```python
from build123d import *

# Parameters (mm, degrees)
ESQUISSE2_W                     = 381
ESQUISSE2_H                     = 95.25
BOSS_EXTRU_1_DEPTH              = 6.35
ESQUISSE3_W                     = 38.1
ESQUISSE3_H                     = 6.35
BOSS_EXTRU_2_DEPTH              = 6.35
ESQUISSE4_W                     = 38.1
ESQUISSE4_H                     = 6.35
ENL_V_MAT_EXTRU_1_DEPTH         = 6.35
R_P_TITION_LIN_AIRE1_COUNT      = 4
R_P_TITION_LIN_AIRE1_PITCH      = 76.2
R_P_TITION_LIN_AIRE1_COUNT_DIR2 = 2
R_P_TITION_LIN_AIRE1_PITCH_DIR2 = 88.9


with BuildPart() as part:
    # Esquisse2 → Boss.-Extru.1 (new body)
    with BuildSketch(Plane(origin=(0, 0, 0), x_dir=(1, 0, 0), z_dir=(0, 1, 0))):
        Rectangle(ESQUISSE2_W, ESQUISSE2_H)
    extrude(amount=BOSS_EXTRU_1_DEPTH)

    # Esquisse3 → Boss.-Extru.2 (add)
    with BuildSketch(Plane(origin=(190.5, 0, 0), x_dir=(0, 0, -1), z_dir=(1, 0, 0))):
        with Locations((0, 3.175)):
            Rectangle(ESQUISSE3_W, ESQUISSE3_H)
    boss_extru_2 = extrude(amount=BOSS_EXTRU_2_DEPTH)

    # Esquisse4 → Enlèv. mat.-Extru.1 (cut)
    with BuildSketch(Plane(origin=(0, 0, -47.625), x_dir=(-1, 0, 0), z_dir=(0, 0, -1))):
        with Locations((-114.3, 3.175)):
            Rectangle(ESQUISSE4_W, ESQUISSE4_H)
    enl_v_mat_extru_1 = extrude(amount=-ENL_V_MAT_EXTRU_1_DEPTH, mode=Mode.SUBTRACT)

    # Répétition linéaire1: Enl_v. mat.-Extru.1 4 × 2
    with Locations(*[(-i * R_P_TITION_LIN_AIRE1_PITCH, 0, j * R_P_TITION_LIN_AIRE1_PITCH_DIR2) for i in range(R_P_TITION_LIN_AIRE1_COUNT) for j in range(R_P_TITION_LIN_AIRE1_COUNT_DIR2) if (i, j) != (0, 0)]):
        add(enl_v_mat_extru_1, mode=Mode.SUBTRACT)

    # Symétrie1: Boss.-Extru.2 across plane
    add(boss_extru_2.mirror(Plane(origin=(0, 0, 0), x_dir=(0, 0, 1), z_dir=(1, 0, 0))))


solid = part.part
```
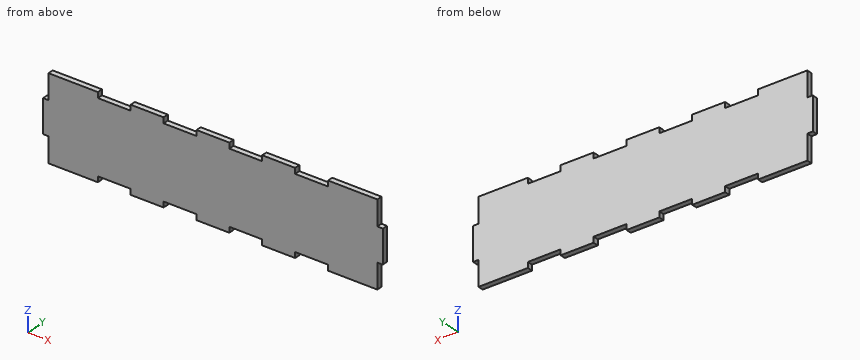
Input: part model. Units: mm. Frame: model coordinates. Give positions to 0.01 mm unless a question says otherwise; leave off trailing zeros. Order: outer loops, then holes, each group sorted by start corner. A loop starts at its lowest first (then second) coordinate and runs counter-clockwise, first axis right, second up. Notation, with made-up numbers: (11, -14.75) - (69, -14.75) arc R9 cw to (69, -0.75) - close; hole circle Ø11 at (-23, 37.25). An arc over 180 degrees is marked (long way). Use a Markdown table: item, result.
(1) Line query: line 1 (X direction, y = 2, z = -38.5); line 2 (Z direction, x = -107, y = 1.25) (3 decimals). Output: solid intervals per line, ascending. Write a range as from..to.
Computed values:
| item | result |
|---|---|
| line 1 | x = -190.5..190.5 |
| line 2 | z = -41.275..41.275 |
(2) Section query A-A (z = 31). Output: boundary loops of the cut face in (x, y).
Computed values:
| item | result |
|---|---|
| outline | (-190.5, 0) - (190.5, 0) - (190.5, 6.35) - (-190.5, 6.35) - close |
(3) Pin query (flat end, axial travel): pin 1 (3 mm diameter, centred on y = 3, z = -43.5, fed in from +X); pin 2 (1.9 mm diameter, centred on y = 4.5, z = 46, fed in from -X); pin 3 (3 mm diameter, centred on x = 114, y = 2, fed in from -Z) (3 decimals). Return the tip coordinate at first contact, or that it passes through.
Computed values:
| item | result |
|---|---|
| pin 1 | stops at x = 190.5 |
| pin 2 | stops at x = -190.5 |
| pin 3 | stops at z = -41.275 |
(4) Section query B-B (x = -27). Output: boundary loops of the cut face in (y, z) (3 decimals), then the cut area to 3 significant figures.
Computed values:
| item | result |
|---|---|
| outline | (0, -41.275) - (6.35, -41.275) - (6.35, 41.275) - (0, 41.275) - close |
| area | 524 mm2 |
